Model file for the job. Use its own axes, mm. A direction names the side the tool comes from. Round coordinates to 2 decimals unless told otherwise and drop trailing zeros. Order: outer loops, then holes, each group sorted by start corner. A loop starts at its lowest first (then second) coordinate and runs counter-clockwise, first axis right, second up. Notation, with made-up numbers: (48.25, -16.75) -> (76.25, -16.75) arc R33 cw to (76.25, 21.25) -> close; hole circle Ø6 at (88, 45). An arc over 180 degrees is marked (long way). Answer as CSV lines item,"result".
```python
from build123d import *

# Parameters (mm, degrees)
SKETCH1_R           = 1.5
BOSS_EXTRUDE1_DEPTH = 8
BOSS_EXTRUDE2_DEPTH = 30
FILLET1_R           = 2
BOSS_EXTRUDE3_DEPTH = 9
SKETCH4_R           = 11
BOSS_EXTRUDE4_DEPTH = 2
SKETCH5_R           = 2.5
BOSS_EXTRUDE5_DEPTH = 22


with BuildPart() as part:
    # Sketch1 → Boss-Extrude1 (new body)
    with BuildSketch(Plane(origin=(0, 0, 0), x_dir=(1, 0, 0), z_dir=(0, 1, 0))):
        Polygon((-17, 21), (17, 21), (21, 17), (21, -17), (17, -21), (-17, -21), (-21, -17), (-21, 17), align=None)
        with Locations(Location((-15.5, 15.5, 0), (0, 0, 270))):
            Circle(SKETCH1_R, mode=Mode.SUBTRACT)
        with Locations(Location((-15.5, -15.5, 0), (0, 0, 270))):
            Circle(SKETCH1_R, mode=Mode.SUBTRACT)
        with Locations(Location((15.5, -15.5, 0), (0, 0, 270))):
            Circle(SKETCH1_R, mode=Mode.SUBTRACT)
        with Locations(Location((15.5, 15.5, 0), (0, 0, 270))):
            Circle(SKETCH1_R, mode=Mode.SUBTRACT)
    extrude(amount=BOSS_EXTRUDE1_DEPTH)

    # Sketch2 → Boss-Extrude2 (add)
    with BuildSketch(Plane.XZ):
        Polygon((-12.75, 20.75), (12.75, 20.75), (20.75, 12.75), (20.75, -12.75), (12.75, -20.75), (-12.75, -20.75), (-20.75, -12.75), (-20.75, 12.75), align=None)
    extrude(amount=BOSS_EXTRUDE2_DEPTH)

    # Fillet1
    fillet1_edges = [part.edges().sort_by_distance(p)[0] for p in [
        (20.75, -15, 12.75),
        (12.75, -15, 20.75),
        (-12.75, -15, 20.75),
        (-20.75, -15, 12.75),
        (-20.75, -15, -12.75),
        (-12.75, -15, -20.75),
        (12.75, -15, -20.75),
        (20.75, -15, -12.75),
    ]]
    fillet(fillet1_edges, radius=FILLET1_R)

    # Sketch3 → Boss-Extrude3 (add)
    with BuildSketch(Plane.XZ.offset(30)):
        Polygon((-21, 17), (-21, -17), (-17, -21), (17, -21), (21, -17), (21, 17), (17, 21), (-17, 21), align=None)
    extrude(amount=BOSS_EXTRUDE3_DEPTH)

    # Sketch4 → Boss-Extrude4 (add)
    with BuildSketch(Plane(origin=(0, 8, 0), x_dir=(1, 0, 0), z_dir=(0, 1, 0))):
        with Locations(Location((0, 0, 0), (0, 0, 90))):
            Circle(SKETCH4_R)
    extrude(amount=BOSS_EXTRUDE4_DEPTH)

    # Sketch5 → Boss-Extrude5 (add)
    with BuildSketch(Plane(origin=(0, 10, 0), x_dir=(1, 0, 0), z_dir=(0, 1, 0))):
        with Locations(Location((0, 0, 0), (0, 0, 270))):
            Circle(SKETCH5_R)
    extrude(amount=BOSS_EXTRUDE5_DEPTH)


solid = part.part
```
Q1. Mould opens along Y. For faces 5 (the flat face through (0, 10, 3)), 6 (the flat face through (0, -34, 21)), 7 (the flat face through (16.8, -14.8, -16.7)) say: +Y half, -Y half, draft (parallel to the pull), parting line (faces both ways), or undercut.
Checks:
face 5,"+Y half"
face 6,"draft"
face 7,"undercut"
Q2. Tool access for faces 1 (the flat face through (0, -15, 20.75)), 2 (the cylindrical face through (-15.43, 3.94, -17)), 3 (the cylindrical face through (12.68, -15.21, -20.6)), 4 (the flat face through (20.75, -15, 0)): list every direction of +Z, -Z, +X, -X, +Y, -Y with a clear straight run to the whole face (end or side of a thin tool).
Checks:
face 1,"+Z, +X, -X"
face 2,"+Y"
face 3,"-Z, +X"
face 4,"+Z, -Z, +X"
Q3. Wall check: L1, parallel to X at y = 5.5, z = 15.5; L2, parallel to Z at x = 15, y = 4; L3, parallel to Y at x = 16, z = 19. Give the ranges that are in metal, low to high. Write a range as [from, to].
Checks:
L1,"[-21, -17], [-14, 14], [17, 21]"
L2,"[-21, -16.91], [-14.09, 14.09], [16.91, 21]"
L3,"[-39, -30], [0, 8]"
Q4. Saw through at A-A (y = -18.5). Write the cut outline in (x, z), plus the area to 3 significant figures.
Checks:
outline,"(-20.75, -11.92) arc R2 ccw to (-20.16, -13.34) -> (-13.34, -20.16) arc R2 ccw to (-11.92, -20.75) -> (11.92, -20.75) arc R2 ccw to (13.34, -20.16) -> (20.16, -13.34) arc R2 ccw to (20.75, -11.92) -> (20.75, 11.92) arc R2 ccw to (20.16, 13.34) -> (13.34, 20.16) arc R2 ccw to (11.92, 20.75) -> (-11.92, 20.75) arc R2 ccw to (-13.34, 20.16) -> (-20.16, 13.34) arc R2 ccw to (-20.75, 11.92) -> close"
area,"1,590 mm²"
Q5. Flat gauge pins, fed straight in: pin 1 (3.5 mm diameter, centred on x = -15, z = -16, fed in from +Y); pin 2 (0.9 mm diameter, centred on x = 16, z = -16, fed in from +Y); pin 3 (12 mm diameter, centred on x = -4.5, z = -2, fed in from +Y); pin 4 (7 mm diameter, centred on x = -1.5, y = -19.5, fed in from +Z). Where does each tip first touch, or does it go through?
Checks:
pin 1,"y = 8"
pin 2,"y = 0"
pin 3,"y = 32"
pin 4,"z = 20.75"
Q6. Saw through at C-C (z = 15.5). Write the cut outline in (x, y), plus the area to 3 significant figures.
Checks:
outline,"(-21, -39) -> (21, -39) -> (21, -30) -> (18, -30) -> (18, 0) -> (21, 0) -> (21, 8) -> (17, 8) -> (17, 0) -> (14, 0) -> (14, 8) -> (-14, 8) -> (-14, 0) -> (-17, 0) -> (-17, 8) -> (-21, 8) -> (-21, 0) -> (-18, 0) -> (-18, -30) -> (-21, -30) -> close"
area,"1,750 mm²"
Q7. Saw through at B-B (x = 0). Write the cut outline in (y, z).
Checks:
outline,"(-39, -21) -> (-30, -21) -> (-30, -20.75) -> (0, -20.75) -> (0, -21) -> (8, -21) -> (8, -11) -> (10, -11) -> (10, -2.5) -> (32, -2.5) -> (32, 2.5) -> (10, 2.5) -> (10, 11) -> (8, 11) -> (8, 21) -> (0, 21) -> (0, 20.75) -> (-30, 20.75) -> (-30, 21) -> (-39, 21) -> close"
Q8. Saw through at D-D (x = -6.5). Write the cut outline in (y, z), plus the area to 3 significant figures.
Checks:
outline,"(-39, -21) -> (-30, -21) -> (-30, -20.75) -> (0, -20.75) -> (0, -21) -> (8, -21) -> (8, -8.87) -> (10, -8.87) -> (10, 8.87) -> (8, 8.87) -> (8, 21) -> (0, 21) -> (0, 20.75) -> (-30, 20.75) -> (-30, 21) -> (-39, 21) -> close"
area,"1,990 mm²"
